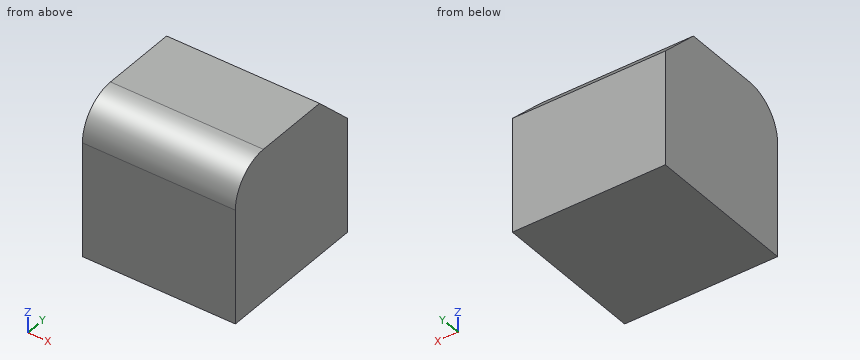
from build123d import *

# Parameters (mm, degrees)
F0_W     = 20
F0_H     = 20
F1_DEPTH = 20
F2_SIZE  = 5
F3_R     = 5


with BuildPart() as f1:
    # F0 (on Top) → F1 (new body)
    with BuildSketch(Plane.XY):
        Rectangle(F0_W, F0_H)
    extrude(amount=F1_DEPTH)

    # F2
    f2_edges = [f1.edges().sort_by_distance(p)[0] for p in [
        (0, 10, 20),
    ]]
    chamfer(f2_edges, length=F2_SIZE)

    # F3
    f3_edges = [f1.edges().sort_by_distance(p)[0] for p in [
        (0, -10, 20),
    ]]
    fillet(f3_edges, radius=F3_R)


solid = f1.part
Model file for the job. Use its own axes, mm. Round coordinates to 2 decimals unless told otherwise and drop trailing zeros. Order: outer loops, then holes, each group sorted by start corner. A loop starts at its lowest first (then second) coordinate and runs counter-clockwise, first axis right, second up.
(1) Band-saw the part on A-A (x = -7). List the corners of the cut face in (y, z).
(2) Pin check, flat tip, straight feed: pin 1 (1 mm diameter, centred on x = 7.5, y = -6, fed in from +Z). Stop position of the tip, or through.
(3) Band-saw the part on C-C (z = 17.5). List the corners of the cut face in (x, y), then the cut area to 3 significant figures.
(4) Drill centre lines: line 1 (Y direction, x = -7.5, z = 17.25); line 2 (Y direction, x = -4.25, z = 15.75); line 3 (Z direction, x = -7.75, y = 5.25). Where is each one in solid material? Low to high.
(5) Band-saw the part on B-B (y = 6.5). List the corners of the cut face in (x, z), then the cut area to 3 significant figures.
Verdict:
1. outline: (-10, 0) - (10, 0) - (10, 15) - (5, 20) - (-5, 20) arc R5 ccw to (-10, 15) - close
2. pin 1: stops at z = 19.97
3. outline: (-10, -9.33) - (10, -9.33) - (10, 7.5) - (-10, 7.5) - close
3. area: 337 mm2
4. line 1: y = -9.47 to 7.75
4. line 2: y = -9.94 to 9.25
4. line 3: z = 0 to 19.75
5. outline: (-10, 0) - (10, 0) - (10, 18.5) - (-10, 18.5) - close
5. area: 370 mm2
